Can you work these out from the model? Positions are in its coordinate system, mm. Face numbers are marked on the shaded views. A direction names the side the tool comes from. Give positions to 0.01 mm unless a question says otherwise; leave off trailing zeros. Loops run counter-clockwise (first coordinate to the right, second up) from the corner with the lowest first, then second, coordinate; pieces in that order, holes last. Notation, with made-up numbers: (-14, 59.25) - (10, 59.25) arc R19 cw to (10, 92.25) - close; hole circle Ø5 at (50, 9). An arc over 180 degrees is marked (long way). Write item = value, one per line.
from build123d import *

# Parameters (mm, degrees)
CYLINDER054_R       = 1.5
CYLINDER054_DEPTH   = 12
ARRAY001025_X_COUNT = 2
ARRAY001025_X_PITCH = 76
ARRAY001025_Y_COUNT = 2
ARRAY001025_Y_PITCH = 26
BOX026_W            = 82
BOX026_H            = 32
BOX026_DEPTH        = 12
BOX025_W            = 86
BOX025_H            = 36
BOX025_DEPTH        = 12
BOX028_W            = 30
BOX028_H            = 20
BOX028_DEPTH        = 10
BOX027_W            = 86
BOX027_H            = 36
BOX027_DEPTH        = 2
CYLINDER053_R       = 4
CYLINDER053_DEPTH   = 12
ARRAY001024_X_COUNT = 2
ARRAY001024_X_PITCH = 76
ARRAY001024_Y_COUNT = 2
ARRAY001024_Y_PITCH = 26


with BuildPart() as obj1:
    # Cylinder054 → Cylinder054 (new body)
    with BuildSketch(Plane(origin=(5, 5, 0), x_dir=(1, 0, 0), z_dir=(0, 0, 1))):
        Circle(CYLINDER054_R)
    extrude(amount=CYLINDER054_DEPTH)

    # Array001025 X: obj1_2


with BuildPart() as obj1_1:
    add(obj1.part)
    with Locations(*[(i * ARRAY001025_X_PITCH, 0, 0) for i in range(1, ARRAY001025_X_COUNT)]):
        add(obj1.part)

    # Array001025 Y: obj1_2


with BuildPart() as obj1_2:
    add(obj1_1.part)
    with Locations(*[(0, i * ARRAY001025_Y_PITCH, 0) for i in range(1, ARRAY001025_Y_COUNT)]):
        add(obj1_1.part)


with BuildPart() as extraction_cube:
    # Box026 → Box026 (new body)
    with BuildSketch(Plane(origin=(2, 2, 0), x_dir=(1, 0, 0), z_dir=(0, 0, 1))):
        with Locations((41, 16)):
            Rectangle(BOX026_W, BOX026_H)
    extrude(amount=BOX026_DEPTH)


with BuildPart() as obj2:
    # Box025 → Box025 (new body)
    with BuildSketch(Plane.XY):
        with Locations((43, 18)):
            Rectangle(BOX025_W, BOX025_H)
    extrude(amount=BOX025_DEPTH)

    # Cut022: cut extraction cube
    add(extraction_cube.part, mode=Mode.SUBTRACT)


with BuildPart() as obj3:
    # Box028 → Box028 (new body)
    with BuildSketch(Plane(origin=(28, 3, -5), x_dir=(1, 0, 0), z_dir=(0, 0, 1))):
        with Locations((15, 10)):
            Rectangle(BOX028_W, BOX028_H)
    extrude(amount=BOX028_DEPTH)


with BuildPart() as obj4:
    # Box027 → Box027 (new body)
    with BuildSketch(Plane.XY):
        with Locations((43, 18)):
            Rectangle(BOX027_W, BOX027_H)
    extrude(amount=BOX027_DEPTH)

    # Cut023002: cut obj3
    add(obj3.part, mode=Mode.SUBTRACT)


with BuildPart() as obj4_1:
    # Cut023002 placement: moved
    add(obj4.part.moved(Location((0, 0, 6.5))))


with BuildPart() as obj5:
    # Cylinder053 → Cylinder053 (new body)
    with BuildSketch(Plane(origin=(5, 5, 0), x_dir=(1, 0, 0), z_dir=(0, 0, 1))):
        Circle(CYLINDER053_R)
    extrude(amount=CYLINDER053_DEPTH)

    # Array001024 X: obj5_2


with BuildPart() as obj5_1:
    add(obj5.part)
    with Locations(*[(i * ARRAY001024_X_PITCH, 0, 0) for i in range(1, ARRAY001024_X_COUNT)]):
        add(obj5.part)

    # Array001024 Y: obj5_2


with BuildPart() as obj5_2:
    add(obj5_1.part)
    with Locations(*[(0, i * ARRAY001024_Y_PITCH, 0) for i in range(1, ARRAY001024_Y_COUNT)]):
        add(obj5_1.part)

    # Fusion035: union obj2, obj4
    add(obj2.part)
    add(obj4_1.part)

    # Cut023: cut obj1
    add(obj1_2.part, mode=Mode.SUBTRACT)


solid = obj5_2.part
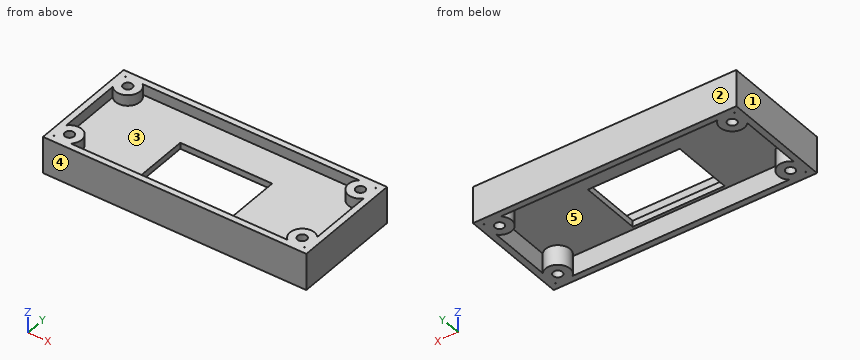
Q1. We'd pull the mould along X, two halves only. Please class the marked faces 1, 2 and 3: released by +X, released by -X, zero draft, split by the parting line, or undercut.
Output:
face_1 = released by -X
face_2 = zero draft
face_3 = undercut
Q2. Imagine slicing it at D-D, the plane z = 3. Give the number of separate pieces and of enclosed holes in the cut face, then the cut area to 3 significant figures.
Output:
separate_pieces = 1
enclosed_holes = 9
area = 616 mm2
Q3. For pin 1 (10 mm diameter, centred on x = 32.5, y = 28, fed in from -Z), with a flat end and sliding along its axis, tell me the tip position at first contact or that it passes through.
Output:
pin_1 = 6.5
Q4. I need wall thicknesses on L1, parallel to Y at x = 5, z = 3.5; L2, parallel to Y at x = 81, z = 8.25; L3, parallel to Y at x = 52, z = 4. Which ranges of each line are inside material? Lowest first, please.
Output:
L1 = 0 to 3.5, 6.5 to 9, 27 to 29.5, 32.5 to 36
L2 = 0 to 3.5, 6.5 to 29.5, 32.5 to 36
L3 = 0 to 2, 34 to 36
Q5. Imagine slicing it at B-B, the plane x = 34.5. Write out the boundary of the cut face in (y, z), then the cut area to 3 significant figures.
Output:
outline = (0, 0) - (2, 0) - (2, 6.5) - (3, 6.5) - (3, 8.5) - (2, 8.5) - (2, 12) - (0, 12) - close; (23, 6.5) - (34, 6.5) - (34, 0) - (36, 0) - (36, 12) - (34, 12) - (34, 8.5) - (23, 8.5) - close
area = 72.0 mm2
Q6. Which directions (+Z, -Z, +X, -X, +Y, -Y) give clear straight access to the entire face, cutting with the end or side of a thin tool? Please do the marked faces 4 and 5.
Output:
face_4 = +Z, -Z, +X, -X, -Y
face_5 = -Z
Q7. Imagine slicing it at C-C, the plane y = 5. Write out the boundary of the cut face in (x, z), then the cut area to 3 significant figures.
Output:
outline = (0, 0) - (3.5, 0) - (3.5, 12) - (0, 12) - close; (6.5, 0) - (9, 0) - (9, 6.5) - (28, 6.5) - (28, 8.5) - (9, 8.5) - (9, 12) - (6.5, 12) - close; (58, 6.5) - (77, 6.5) - (77, 0) - (79.5, 0) - (79.5, 12) - (77, 12) - (77, 8.5) - (58, 8.5) - close; (82.5, 0) - (86, 0) - (86, 12) - (82.5, 12) - close
area = 220 mm2
Q8. Imagine slicing it at A-A, the plane y = 31. Write out the boundary of the cut face in (x, z).
Output:
outline = (0, 0) - (3.5, 0) - (3.5, 12) - (0, 12) - close; (6.5, 0) - (9, 0) - (9, 6.5) - (77, 6.5) - (77, 0) - (79.5, 0) - (79.5, 12) - (77, 12) - (77, 8.5) - (9, 8.5) - (9, 12) - (6.5, 12) - close; (82.5, 0) - (86, 0) - (86, 12) - (82.5, 12) - close
